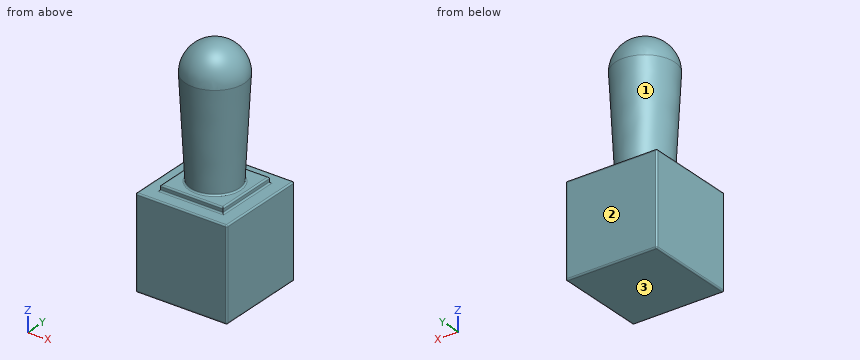
```python
from build123d import *

# Parameters (mm, degrees)
F0_W     = 32
F0_H     = 32
F1_DEPTH = 32
F2_W     = 22
F2_H     = 22
F3_DEPTH = 2
F4_R     = 8.5
F5_DEPTH = 35
F5_TAPER = -3
F8_R     = 0.5
F9_R     = 0.5


with BuildPart() as f1:
    # F0 (on Top) → F1 (new body)
    with BuildSketch(Plane.XY):
        Rectangle(F0_W, F0_H)
    extrude(amount=F1_DEPTH)

    # F2 (on face) → F3 (join)
    with BuildSketch(Plane.XY.offset(32)):
        Rectangle(F2_W, F2_H)
    extrude(amount=F3_DEPTH)

    # F4 (on face) → F5 (join)
    with BuildSketch(Plane.XY.offset(34)):
        Circle(F4_R)
    extrude(amount=F5_DEPTH, taper=F5_TAPER)

    # F6 (on face) → F7 (revolve)
    with BuildSketch(Plane.XY.offset(69)):
        with BuildLine():
            ThreePointArc((10.3342722749, 0), (0, 10.3342722749), (-10.3342722749, 0))
            Line((-10.3342722749, 0), (0, 0))
            Line((0, 0), (10.3342722749, 0))
        make_face()
    revolve(axis=Axis((-5.1671361375, 0, 69), (1, 0, 0)))

    # F8
    f8_edges = [f1.edges().sort_by_distance(p)[0] for p in [
        (0, -11, 34),
        (11, 0, 34),
        (11, 0, 32),
        (0, -11, 32),
        (0, 16, 0),
        (0, 11, 32),
        (0, 11, 34),
        (-11, 0, 32),
        (-11, 0, 34),
        (-8.5, 0, 34),
    ]]
    fillet(f8_edges, radius=F8_R)

    # F9
    f9_edges = [f1.edges().sort_by_distance(p)[0] for p in [
        (0, -16, 32),
        (16, 0, 32),
        (16, -16, 16),
        (16, 16, 16.25),
        (-16, -16, 16),
        (0, -16, 0),
        (16, -0.25, 0),
        (0, 16, 32),
        (-16, 0, 32),
        (-16, -0.25, 0),
    ]]
    fillet(f9_edges, radius=F9_R)


solid = f1.part
```
Could you check a few things on this model? Use its own coordinates, in mm. Face numbers are marked on the shaded views. Round coordinates to 2 decimals unless told otherwise and drop trailing zeros. Loops run counter-clockwise (first coordinate to the right, second up) from the corner with the lowest first, then second, coordinate; pieces in that order, holes last. Notation, with made-up numbers: (-14.5, 50) - (25.5, 50) arc R22 ccw to (25.5, 87) - close; hole circle Ø10 at (26, 73). An arc over 180 degrees is marked (long way). Answer as CSV lines item,"result".
1. Please list where these lines run through material, in increasing order: line 1 along Z through (x, y) = (12.5, -13); line 2 along Z through (x, y) = (9, 9.5); line 3 along Y through (x, z) = (5.5, 66.5). Write a range as [from, to].
Filled in:
line 1,"z = [0, 32]"
line 2,"z = [0, 34]"
line 3,"y = [-8.59, 8.59]"
2. For pin 1 Ø2 at (x, z) = (-5.5, 70) entering from +Y; pin 2 Ø2 at (y, z) = (-8.5, 36.5) entering from -X; pin 3 Ø0.8 at (y, z) = (3.5, 33) entering from -X, each with a flat end and sliding along its axis, tell me the tip position at first contact or that it passes through.
Filled in:
pin 1,"stops at y = 9.26"
pin 2,"stops at x = -4.27"
pin 3,"stops at x = -11"
3. I want a section at A-A on y = 13. List the corners of the cut face in (x, z) for me.
Filled in:
outline,"(-16, 0.5) arc R0.5 ccw to (-15.5, 0) - (15.5, 0) arc R0.5 ccw to (16, 0.5) - (16, 31.5) arc R0.5 ccw to (15.5, 32) - (-15.5, 32) arc R0.5 ccw to (-16, 31.5) - close"
4. I want a section at B-B on x = 0. List the corners of the cut face in (y, z) for me, then the cut area to 3 significant figures.
Filled in:
outline,"(-16, 0.5) arc R0.5 ccw to (-15.5, 0) - (15.5, 0) arc R0.5 ccw to (16, 0.5) - (16, 31.5) arc R0.5 ccw to (15.5, 32) - (11.5, 32) arc R0.5 cw to (11, 32.5) - (11, 33.5) arc R0.5 ccw to (10.5, 34) - (9.03, 34) arc R0.5 cw to (8.53, 34.53) - (10.33, 69) arc R10.33 ccw to (-10.33, 69) - (-8.53, 34.53) arc R0.5 cw to (-9.03, 34) - (-10.5, 34) arc R0.5 ccw to (-11, 33.5) - (-11, 32.5) arc R0.5 cw to (-11.5, 32) - (-15.5, 32) arc R0.5 ccw to (-16, 31.5) - close"
area,"1,890 mm^2"
5. We'd pull the mould along Z, two halves only. Please class the marked faces 1, 2 and 3: +Z half, -Z half, draft (parallel to the pull), parting line (faces both ways), or undercut.
Filled in:
face 1,"undercut"
face 2,"draft"
face 3,"-Z half"
6. I want a section at C-C on z = 49.5. List the corners of the cut face in (x, y) for me.
Filled in:
outline,"circle Ø18.62 at (0, 0)"
